For this review, take the finished solid that the model builds, in its own axes (mm). Coordinates: 2 decimals unless noted, no trailing zeros. Loops run counter-clockwise (first coordinate to the right, second up) from the corner with the lowest first, then second, coordinate; pieces in that order, holes last. Notation, with made-up numbers: (-38, 86) - (-16, 86) arc R27 ccw to (-16, 108) - close; hole circle Ø10 at (81.25, -16). An arc over 180 degrees is marked (long way). One line per item, written item: value. Start each with the question number.
1. To check wall thickness, follow line 1 (Z direction, x = 13.25, y = 177); line 2 (Y direction, x = 14.75, z = -173); line 3 (Y direction, x = 1.25, z = 141). State the ranges of each line that lie inside material, in increasing order. Write a range as from..to.
2. Insertion check: pin 1 (4 mm diameter, centred on x = 3, z = -86, fed in from -Y); pin 2 (5 mm diameter, centred on x = 9.5, z = 78, fed in from +Y); pin 3 (2.5 mm diameter, centred on x = 3.5, y = -58.5, fed in from +Z). Each pin has a flat end and moves straight along its axis. Give the tip position at first contact, or say it passes through.
3. Take a section at C-C, the plane x = 3. State the section outline as (y, z) points.
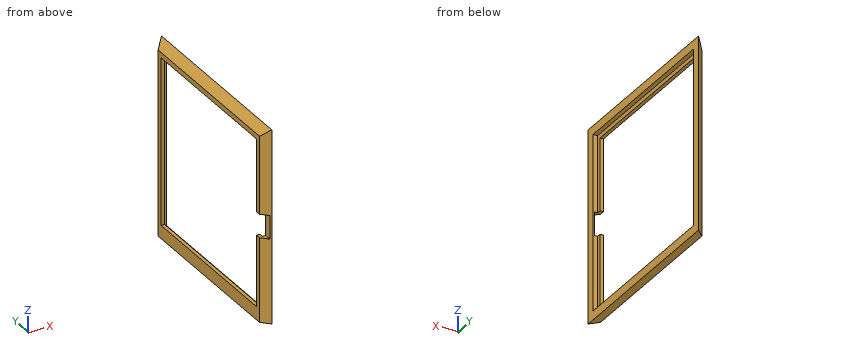
Autodesk Inventor part; units mm, degrees
ref_plane "YZ Plane" through (0, 0, 0) normal (1, 0, 0) x (0, 1, 0)
ref_plane "XZ Plane" through (0, 0, 0) normal (0, 1, 0) x (-1, 0, 0)
ref_plane "XY Plane" through (0, 0, 0) normal (0, 0, 1) x (1, 0, 0)
sketch "Skizze1" plane through (0, 0, 0) normal (1, 0, 0) x (0, 1, 0)
  line L0 (-230.3873, 208.9718) -> (209.6127, 208.9718)
  line L1 (209.6127, 208.9718) -> (209.6127, -231.0282)
  line L2 (209.6127, -231.0282) -> (-230.3873, -231.0282)
  line L3 (-230.3873, -231.0282) -> (-230.3873, 208.9718)
  point P0 (0, 0)
  dimension "d0" = 440
  dimension "d1" = 440
extrude "Extrusion1" add sketch "Skizze1" along normal blind 18
sketch "Skizze2" plane through (18, 0, 0) normal (1, 0, 0) x (0, 0, -1)
  line L0 (-208.9718, 209.6127) -> (-208.9718, -230.3873)
  line L1 (-208.9718, -230.3873) -> (231.0282, -230.3873)
  line L2 (231.0282, -230.3873) -> (231.0282, 209.6127)
  line L3 (231.0282, 209.6127) -> (-208.9718, 209.6127)
  line L4 (-188.9718, -210.3873) -> (211.0282, -210.3873)
  line L5 (211.0282, -210.3873) -> (211.0282, 189.6127)
  line L6 (211.0282, 189.6127) -> (-188.9718, 189.6127)
  line L7 (-188.9718, 189.6127) -> (-188.9718, -210.3873)
  point P0 (0, 0)
  dimension "d4" = 20
  dimension "d5" = 20
  dimension "d6" = 20
  dimension "d7" = 20
extrude "Extrusion2" cut sketch "Skizze2" against normal blind 10 contours L7 L6 L5 L4
sketch "Skizze3" plane through (8, 0, 0) normal (1, 0, 0) x (0, 0, -1)
  line L0 (211.0282, -210.3873) -> (-188.9718, -210.3873)
  line L1 (211.0282, 189.6127) -> (211.0282, -210.3873)
  line L2 (-188.9718, 189.6127) -> (211.0282, 189.6127)
  line L3 (-188.9718, -210.3873) -> (-188.9718, 189.6127)
  line L4 (-178.9718, -200.3873) -> (201.0282, -200.3873)
  line L5 (201.0282, -200.3873) -> (201.0282, 179.6127)
  line L6 (201.0282, 179.6127) -> (-178.9718, 179.6127)
  line L7 (-178.9718, 179.6127) -> (-178.9718, -200.3873)
  point P0 (0, 0)
  dimension "d10" = 10
  dimension "d11" = 10
  dimension "d12" = 10
  dimension "d13" = 10
extrude "Extrusion3" cut sketch "Skizze3" against normal blind 8 contours L7 L6 L5 L4
sketch "Skizze6" plane through (0, 0, 0) normal (-1, 0, 0) x (0, 0, 1)
  line L0 (-201.0282, -200.3873) -> (-201.0282, 179.6127)
  line L1 (-201.0282, 179.6127) -> (178.9718, 179.6127)
  line L2 (178.9718, 179.6127) -> (178.9718, -200.3873)
  line L3 (178.9718, -200.3873) -> (-201.0282, -200.3873)
  line L4 (208.9718, -230.3873) -> (208.9718, 209.6127)
  line L5 (208.9718, 209.6127) -> (-231.0282, 209.6127)
  line L6 (-231.0282, 209.6127) -> (-231.0282, -230.3873)
  line L7 (-231.0282, -230.3873) -> (208.9718, -230.3873)
  line L8 (6.4718, -214.3873) -> (6.4718, -223.3873)
  line L9 (10.9718, -214.3873) -> (6.4718, -214.3873)
  line L10 (6.4718, -223.3873) -> (1.9718, -223.3873)
  line L11 (1.9718, -210.3873) -> (1.9718, -223.3873)
  line L12 (10.9718, -210.3873) -> (10.9718, -214.3873)
  line L13 (-211.0282, -210.3873) -> (188.9718, -210.3873)
  line L14 (-0.0282, -210.3873) -> (-0.0282, -223.3873)
  line L15 (-9.0282, -210.3873) -> (-9.0282, -214.3873)
  line L16 (-4.5282, -214.3873) -> (-9.0282, -214.3873)
  line L17 (-4.5282, -214.3873) -> (-4.5282, -223.3873)
  line L18 (-0.0282, -223.3873) -> (-4.5282, -223.3873)
  line L19 (-16.0282, -210.3873) -> (-16.0282, -214.3873)
  line L20 (-16.0282, -214.3873) -> (-20.5282, -214.3873)
  line L21 (-20.5282, -214.3873) -> (-20.5282, -223.3873)
  line L22 (-20.5282, -223.3873) -> (-25.0282, -223.3873)
  line L23 (-25.0282, -210.3873) -> (-25.0282, -223.3873)
  line L24 (-27.0282, -210.3873) -> (-27.0282, -223.3873)
  line L25 (-27.0282, -223.3873) -> (-31.5282, -223.3873)
  line L26 (-31.5282, -214.3873) -> (-31.5282, -223.3873)
  line L27 (-31.5282, -214.3873) -> (-36.0282, -214.3873)
  line L28 (-36.0282, -210.3873) -> (-36.0282, -214.3873)
  line L29 (-231.0282, -230.3873) -> (208.9718, -230.3873)
  line L30 (14.0665, -230.3873) -> (14.0665, -200.3873)
  line L31 (-39.201, -230.3873) -> (-39.201, -200.3873)
  point P0 (0, 0)
extrude "Extrusion4" cut sketch "Skizze6" against normal blind 15 contours L3 L30 L13 L31 | L13 L28 L27 L26 L25 L24 L23 L22 L21 L20 L19 L15 L16 L17 L18 L14 L11 L10 L8 L9 L12 L30 L7 L31 | L13 L24 L25 L26 L27 L28 | L12 L9 L8 L10 L11 L13 | L13 L19 L20 L21 L22 L23 | L14 L18 L17 L16 L15 L13
chamfer "Fase1" distance 18 angle 45 1 edges at (0, -230.3873, 111.5191)
chamfer "Fase2" distance 18 angle 45 2 edges at (0, 209.6127, -11.0282) (0, -1.3876, 208.9718)
properties part number "PV_Rahmen_CPY"
Solutions:
1. line 1: -231.03..-211.03, 188.97..204.22
1. line 2: -227.14..-210.39, 189.61..206.36
1. line 3: -213.64..-200.39, 179.61..192.86
2. pin 1: y = -217.39
2. pin 2: y = 203.61
2. pin 3: z = 195.72
3. outline: (-215.39, -231.03) - (194.61, -231.03) - (194.61, 193.97) - (-215.39, 193.97) - (-215.39, 14.07) - (-200.39, 14.07) - (-200.39, 178.97) - (179.61, 178.97) - (179.61, -201.03) - (-200.39, -201.03) - (-200.39, -39.2) - (-215.39, -39.2) - close
